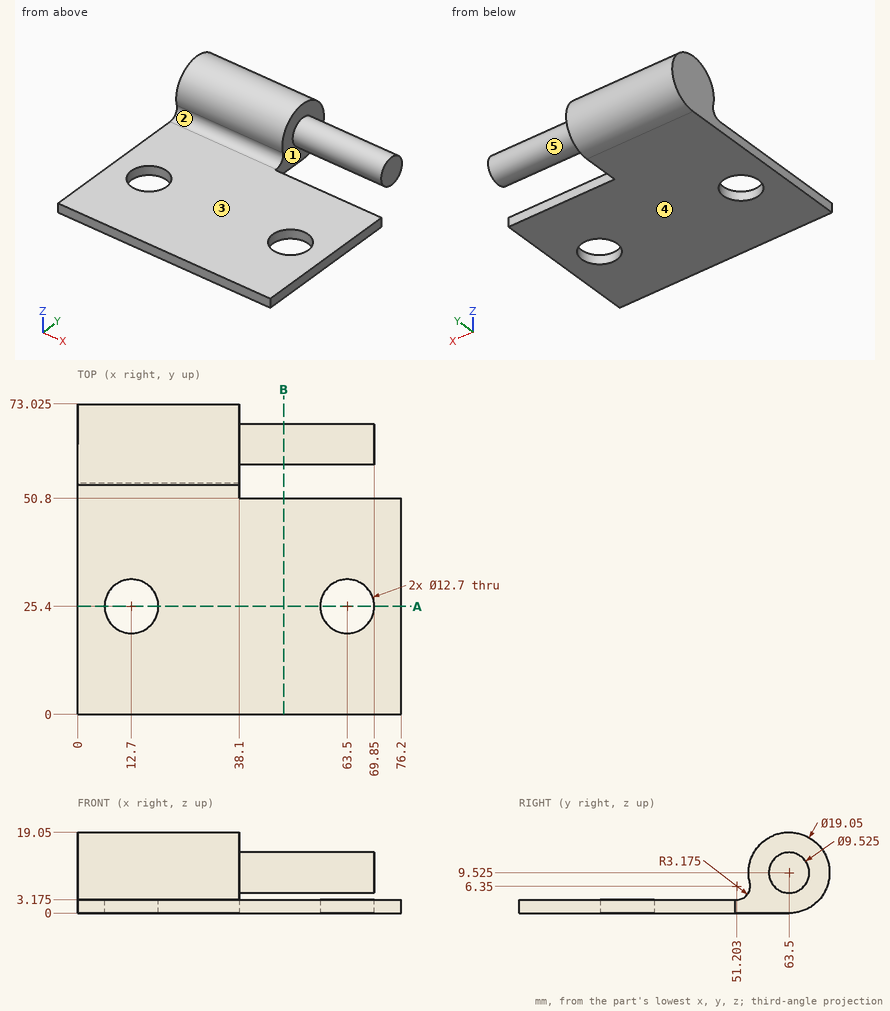
Can you work these out from the drawing? Everything is in mm from the part's minimum corner. A direction names the side the tool comes from. Give positions to 0.01 mm unless a question says otherwise; leave off trailing zeros. Write each loop counter-clockwise with the first axis right and the second up, starting at its lowest first coordinate (ties: lowest second). Pieces come first, ordered by that corner, then holes. Notation, with made-up numbers: (50.5, 78) -> (72.5, 78) arc R23 ccw to (72.5, 93) -> close; hole circle Ø3 at (-33, 51). An arc over 180 degrees is marked (long way). Write each question's results on one line, items separated by ' | '.
Item 1: If I drill on L1, parallel to Y at x = 63.5, z = 2.1; L2, parallel to Z at x = 4, y = 26.5 (1 decimal); L3, parallel to Y at x = 13.5, z = 1.25 (1 decimal), over which ranges is the centre line in solid material (lowest first)?
Output:
L1: y = 0 to 19.05, 31.75 to 50.8 | L2: z = 0 to 3.2 | L3: y = 0 to 19.1, 31.7 to 68.2
Item 2: We'd pull the mould along Z, two halves only. Please class the marked faces 1, 2 and 3: pulls with the +Z half, pulls with the -Z half, needs draft (parallel to the pull), parting line crosses it, or undercut.
Output:
face 1: needs draft | face 2: undercut | face 3: pulls with the +Z half
Item 3: On a 3-axis mill with a long thin cutter (end or side, diameter ignored), from which of +Z, -Z, +X, -X, +Y, -Y can I reach the whole of each face in a straight line? I mean the marked faces 4 and 5. Say none if no direction works.
Output:
face 4: -Z, +X, -X, +Y, -Y | face 5: +X
Item 4: Suppose I cut it at A-A on y = 25.4. Give the number of separate pieces and of enclosed holes in the cut face, plus the area to 3 significant figures.
Output:
separate pieces: 3 | enclosed holes: 0 | area: 161 mm^2
Item 5: Suppose I cut it at B-B on x = 48.5. Write out the boundary of the cut face in (y, z) (1 decimal).
Output:
outline: (0, 0) -> (50.8, 0) -> (50.8, 3.2) -> (0, 3.2) -> close; circle Ø9.5 at (63.5, 9.5)
Item 6: For pin 1 Ø3.5 at (x, z) = (51, 2) entering from +Y; pin 2 Ø5.5 at (y, z) = (67, 12) entering from +X; pin 3 Ø16.5 at (x, y) = (63.5, 25.4) entering from +Z (3 decimals), each with a flat end and sliding along its axis, tell me the tip position at first contact or that it passes through.
Output:
pin 1: stops at y = 50.8 | pin 2: stops at x = 69.85 | pin 3: stops at z = 3.175
